Geometry: see drawing. Coordinates: mm, zero at the bounding-box minimum. A direction names the side the tool comes from. Give positions to 0.01 mm unless a question says otherwise; leave off trailing zeros. Loops run counter-clockwise (first coordinate to the right, second up) from the corner with the lowest first, then second, coordinate; pieces in that order, holes last. Notation, with made-up numbers: M 71,84.25 L 99,84.25 A23 ccw 99,108.25 Z; hole C 80.25,-33.75 d1. An arc over 180 degrees is marked long. Use a Markdown table: item, result. Add a question column.
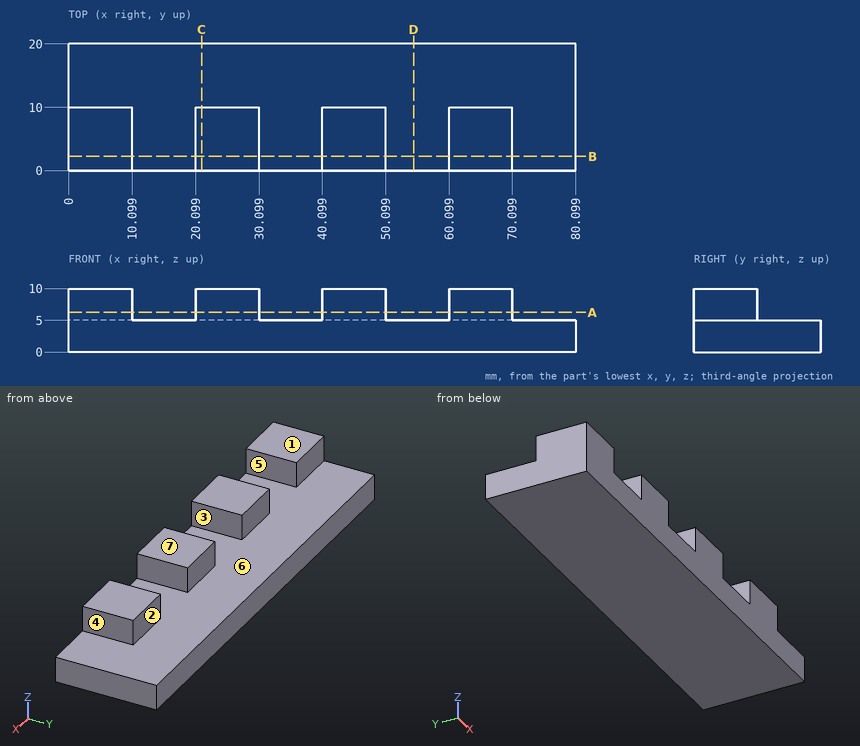
1) Pull-direction query (X, two-part tool) for the marked faces 4, 5, 6 and 7; classes: pulls with the +X half, pulls with the -X half, needs draft (parallel to the pull), parting line crosses it, or undercut.
2) Section query C-C, the plane x = 21. Return the cut outline in (y, z).
3) Contact query for flat-ended pins moving along their axis: P1, Ø5.5, axis at x = 66, z = 8, coming from the +Y side; P2, Ø2.5, axis at y = 5, z = 8.5, coming from the +X side; P3, Ø4, axis at x = 15.5, z = 8.5, coming from the -Y side. Output: stop coordinate, or through.
4) Section query B-B, the plane y = 2.25. Return the cut outline in (x, z).
5) Section query A-A, the plane z = 6.25. Return the cut outline in (x, y).
6) Ray query, line 1 (X direction, y = 8, z = 5.25); line 2 (Z direction, x = 62.5, y = 19); line 3 (Y direction, x = 6, z = 9.25). Return the intervals inside material, ascending. Write a range as [from, to].
7) Section query D-D, the plane x = 54.5. Return the cut outline in (y, z).
8) Reachability of the marked faces 1, 2 and 3 from +Z, -Z, +X, -X, +Y, -Y: full face, straight path, thin tool, end or side. Return the list, or none.
Entries:
| question | item | result |
|---|---|---|
| 1 | face 4 | pulls with the +X half |
| 1 | face 5 | undercut |
| 1 | face 6 | undercut |
| 1 | face 7 | needs draft |
| 2 | outline | M 0,0 L 20,0 L 20,5 L 10,5 L 10,10 L 0,10 Z |
| 3 | P1 | stops at y = 10 |
| 3 | P2 | stops at x = 70.1 |
| 3 | P3 | passes through |
| 4 | outline | M 0,0 L 80.1,0 L 80.1,5 L 70.1,5 L 70.1,10 L 60.1,10 L 60.1,5 L 50.1,5 L 50.1,10 L 40.1,10 L 40.1,5 L 30.1,5 L 30.1,10 L 20.1,10 L 20.1,5 L 10.1,5 L 10.1,10 L 0,10 Z |
| 5 | outline | M 0,0 L 10.1,0 L 10.1,10 L 0,10 Z; M 20.1,0 L 30.1,0 L 30.1,10 L 20.1,10 Z; M 40.1,0 L 50.1,0 L 50.1,10 L 40.1,10 Z; M 60.1,0 L 70.1,0 L 70.1,10 L 60.1,10 Z |
| 6 | line 1 | x = [0, 10.1], [20.1, 30.1], [40.1, 50.1], [60.1, 70.1] |
| 6 | line 2 | z = [0, 5] |
| 6 | line 3 | y = [0, 10] |
| 7 | outline | M 0,0 L 20,0 L 20,5 L 0,5 Z |
| 8 | face 1 | +Z, +X, -X, +Y, -Y |
| 8 | face 2 | +Z, +X, -X, +Y |
| 8 | face 3 | +Z, +Y, -Y |
